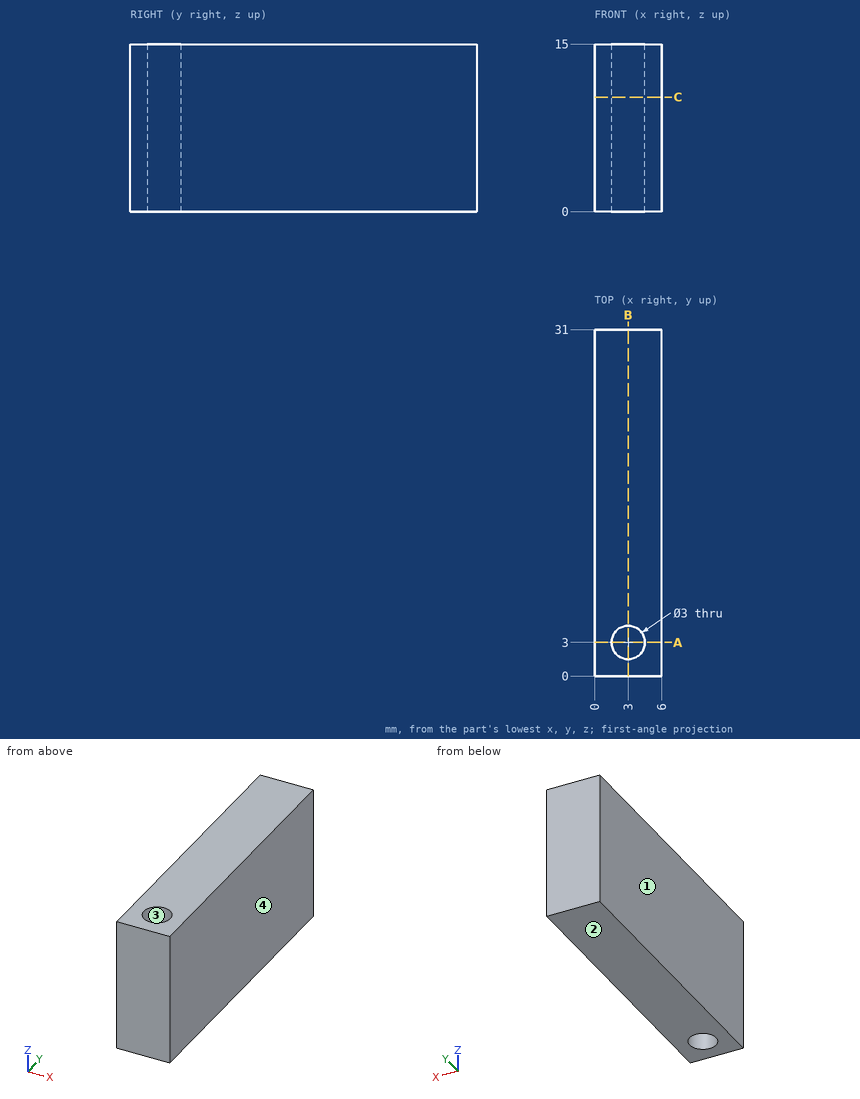
Answer from the drawing. Dimensions are ordinates in mm from the lowest x, y and z of the part. Give positions to 0.01 mm unless a question says otherwise; leave off trailing zeros. Order: outer loops, then holes, each group sorted by start corner. A loop starts at its lowest first (then second) coordinate and runs counter-clockwise, first axis right, second up.
(1) Find section B-B (x = 3). Give the vertices of the cut face in (y, z).
(2) Find section C-C (z = 10.25). Give the vertices of the cut face in (x, y), plus the area to 3 significant figures.
(3) For a pull along X with two mould halves and no side action, classify the marked faces 1, 2, 3 and 4 as released by +X, released by -X, zero draft, split by the parting line, or undercut.
(4) Straight lines are drawn through the part: L1, parallel to Y at x = 3, z = 10.75; L2, parallel to X at y = 3, z = 3.75; L3, parallel to X at y = 4, z = 2.25. For each, find the intervals that lie inside material, in ascending order.
(5) Find section A-A (y = 3). Give the vertices of the cut face in (x, z), plus the area to 3 significant figures.
Result sheet:
1. outline: (0, 0) - (1.5, 0) - (1.5, 15) - (0, 15) - close; (4.5, 0) - (31, 0) - (31, 15) - (4.5, 15) - close
2. outline: (0, 0) - (6, 0) - (6, 31) - (0, 31) - close; hole circle Ø3 at (3, 3)
2. area: 179 mm2
3. face 1: released by -X
3. face 2: zero draft
3. face 3: undercut
3. face 4: released by +X
4. L1: y = 0 to 1.5, 4.5 to 31
4. L2: x = 0 to 1.5, 4.5 to 6
4. L3: x = 0 to 1.88, 4.12 to 6
5. outline: (0, 0) - (1.5, 0) - (1.5, 15) - (0, 15) - close; (4.5, 0) - (6, 0) - (6, 15) - (4.5, 15) - close
5. area: 45.0 mm2
